```python
from build123d import *

# Parameters (mm, degrees)
F0_W     = 69.85
F0_H     = 38.1
F1_DEPTH = 25.4
F3_DEPTH = 25.4
F5_DEPTH = 12.7
F7_DEPTH = 25.4
F8_R     = 6.35
F9_DEPTH = 25.4


with BuildPart() as f1:
    # F0 (on Front) → F1 (new body)
    with BuildSketch(Plane.XZ):
        with Locations((34.925, 19.05)):
            Rectangle(F0_W, F0_H)
    extrude(amount=F1_DEPTH)

    # F2 (on face) → F3 (cut)
    with BuildSketch(Plane.XZ.offset(25.4)):
        with BuildLine():
            Line((0, 38.1), (0, 25.4))
            ThreePointArc((0, 25.4), (3.7197438789, 34.3802561211), (12.7, 38.1))
            Line((12.7, 38.1), (0, 38.1))
        make_face()
        with BuildLine():
            Line((69.85, 38.1), (12.7, 38.1))
            ThreePointArc((12.7, 38.1), (21.6802561211, 34.3802561211), (25.4, 25.4))
            Line((25.4, 25.4), (25.4, 12.7))
            Line((25.4, 12.7), (69.85, 12.7))
            Line((69.85, 12.7), (69.85, 38.1))
        make_face()
    extrude(amount=-F3_DEPTH, mode=Mode.SUBTRACT)

    # F4 (on face) → F5 (join)
    with BuildSketch(Plane.XY.offset(12.7)):
        with BuildLine():
            Line((69.85, -25.4), (82.55, -25.4))
            ThreePointArc((82.55, -25.4), (95.25, -12.7), (82.55, 0))
            Line((82.55, 0), (69.85, 0))
            Line((69.85, 0), (69.85, -25.4))
        make_face()
    extrude(amount=-F5_DEPTH)

    # F6 (on face) → F7 (cut)
    with BuildSketch(Plane.XY.offset(12.7)):
        with BuildLine():
            ThreePointArc((38.0759369288, -5.5685763133), (42.5660649893, -7.4284482528), (44.4259369288, -11.9185763133))
            ThreePointArc((44.4259369288, -11.9185763133), (42.5946024122, -16.3799844149), (38.1569094488, -18.2680600287))
            Line((38.1569094488, -18.2680600287), (57.1243946492, -18.0261748455))
            ThreePointArc((57.1243946492, -18.0261748455), (50.7749087424, -11.7569753348), (56.9628067538, -5.328231135))
            Line((56.9628067538, -5.328231135), (38.0759369288, -5.5685763133))
        make_face()
        with BuildLine():
            Line((57.1243946492, -5.3261748455), (56.9628067538, -5.328231135))
            ThreePointArc((56.9628067538, -5.328231135), (50.7749087424, -11.7569753348), (57.1243946492, -18.0261748455))
            ThreePointArc((57.1243946492, -18.0261748455), (61.6145227098, -16.1663029061), (63.4743946492, -11.6761748455))
            ThreePointArc((63.4743946492, -11.6761748455), (61.6145227098, -7.186046785), (57.1243946492, -5.3261748455))
        make_face()
        with BuildLine():
            ThreePointArc((38.1569094488, -18.2680600287), (42.5946024122, -16.3799844149), (44.4259369288, -11.9185763133))
            ThreePointArc((44.4259369288, -11.9185763133), (42.5660649893, -7.4284482528), (38.0759369288, -5.5685763133))
            ThreePointArc((38.0759369288, -5.5685763133), (31.7260660012, -11.9590633963), (38.1569094488, -18.2680600287))
        make_face()
    extrude(amount=-F7_DEPTH, mode=Mode.SUBTRACT)

    # F8 (on face) → F9 (cut)
    with BuildSketch(Plane.XZ.offset(25.4)):
        with Locations((12.7, 25.4)):
            Circle(F8_R)
    extrude(amount=-F9_DEPTH, mode=Mode.SUBTRACT)


solid = f1.part
```
Design review of the part built by this model. Coordinates are the model's own, in mm. A direction names the side the tool comes from. Give positions to 0.01 mm unless a question says otherwise; leave off trailing zeros. Order: outer loops, then holes, each group sorted by start corner. A loop starts at its lowest first (then second) coordinate and runs counter-clockwise, first axis right, second up. Notation, with made-up numbers: (-29, 2) -> (20, 2) arc R22 cw to (20, 37) -> close; hole circle Ø9 at (-34, -40). An arc over 180 degrees is marked (long way). Write item = value, one per line. Start each with the question number.
(1) For pin 1 (12.5 mm diameter, centred on x = 51, y = -12, fed in from +Z); pin 2 (14 mm diameter, centred on y = -18.5, z = 17.5, fed in from +X); pin 3 (12 mm diameter, centred on y = -21.5, z = 7, fed in from +X), all flat-tipped, find the tip position at first contact; note any pin that passes through.
(2) For faces 1 (the face through (25.4, -13, 19)), 2 (the face through (47, -21, 0)), list the 3-axis set-ups (+Z, -Z, +X, -X, +Y, -Y) from which the entire face can be reached by the end or side of a thin tool; tool diameter is ignored.
(3) We need section D-D on y = -6.75. Write out the cut boundary in (x, z), plus the area to 3 significant figures.
(4) To check wall thickness, follow line 1 along Z through (x, y) = (12.7, -5.25); line 2 along Z through (x, y) = (25.5, -7); line 3 along X through (y, z) = (-16.5, 10). State the ranges of each line that lie inside material, in increasing order.
(5) We need section B-B on z = 4. Write out the cut boundary in (x, y).
(6) We need section A-A on y = -12.7. Write out the cut boundary in (x, z), plus the area to 3 significant figures.
(7) Mouldability with a two-part tool opening along X and no side actions: class faces 3 (the face through (31.727, -11.819, 6.439)), 4 (the face through (7.66, -12.88, 21.54)), 5 (the face through (0, -13, 13)), 6 (the face through (33, 0, 11)) as +X half, -X half, draft (parallel to the pull), parting line (faces both ways), or undercut.
(8) We need section C-C on x = 45. Write out the cut boundary in (y, z), plus the area to 3 significant figures.
Numbers:
q1.pin_1 = 12.7
q1.pin_2 = 95.23
q1.pin_3 = 94.94
q2.face_1 = +Z, +X, +Y, -Y
q2.face_2 = -Z, +X, -X, +Y, -Y
q3.outline = (0, 0) -> (34.39, 0) -> (34.39, 12.7) -> (25.4, 12.7) -> (25.4, 25.4) arc R12.7 ccw to (0, 25.4) -> close; (61.13, 0) -> (93.77, 0) -> (93.77, 12.7) -> (61.13, 12.7) -> close; hole circle Ø12.7 at (12.7, 25.4)
q3.area = 1,300 mm^2
q4.line_1 = 0 to 19.05, 31.75 to 38.1
q4.line_2 = 0 to 12.7
q4.line_3 = 0 to 33.68, 61.25 to 94.67
q5.outline = (0, -25.4) -> (82.55, -25.4) arc R12.7 ccw to (82.55, 0) -> (0, 0) -> close; hole (38.08, -5.57) arc R6.35 ccw (long way) to (38.16, -18.27) -> (57.12, -18.03) arc R6.35 ccw to (57.12, -5.33) -> close
q6.outline = (0, 0) -> (31.77, 0) -> (31.77, 12.7) -> (25.4, 12.7) -> (25.4, 25.4) arc R12.7 ccw to (0, 25.4) -> close; (63.39, 0) -> (95.25, 0) -> (95.25, 12.7) -> (63.39, 12.7) -> close; hole circle Ø12.7 at (12.7, 25.4)
q6.area = 1,260 mm^2
q7.face_3 = undercut
q7.face_4 = undercut
q7.face_5 = -X half
q7.face_6 = draft
q8.outline = (-25.4, 0) -> (-18.18, 0) -> (-18.18, 12.7) -> (-25.4, 12.7) -> close; (-5.48, 0) -> (0, 0) -> (0, 12.7) -> (-5.48, 12.7) -> close
q8.area = 161 mm^2
